```python
from build123d import *

# Parameters (mm, degrees)
SKETCH1_W            = 90
SKETCH1_H            = 70
BOSS_EXTRUDE1_DEPTH  = 10
FILLET1_R            = 4
SHELL1_T             = -2
SKETCH2_W            = 1
SKETCH2_H            = 15
BOSS_EXTRUDE2_DEPTH  = 1
SKETCH3_W            = 0.9
SKETCH3_H            = 15
BOSS_EXTRUDE3_DEPTH  = 0.9
SKETCH4_W            = 0.8
SKETCH4_H            = 15
BOSS_EXTRUDE4_DEPTH  = 0.8
SKETCH5_W            = 0.7
SKETCH5_H            = 15
BOSS_EXTRUDE5_DEPTH  = 0.7
SKETCH6_W            = 0.6
SKETCH6_H            = 15
BOSS_EXTRUDE6_DEPTH  = 0.6
SKETCH7_W            = 0.5
SKETCH7_H            = 15
BOSS_EXTRUDE7_DEPTH  = 0.5
SKETCH8_W            = 0.4
SKETCH8_H            = 15
BOSS_EXTRUDE8_DEPTH  = 0.4
SKETCH9_W            = 0.3
SKETCH9_H            = 15
BOSS_EXTRUDE9_DEPTH  = 0.3
SKETCH10_W           = 0.2
SKETCH10_H           = 15
BOSS_EXTRUDE10_DEPTH = 0.2
SKETCH11_W           = 0.1
SKETCH11_H           = 15
BOSS_EXTRUDE11_DEPTH = 0.1
SKETCH12_W           = 0.075
SKETCH12_H           = 15
BOSS_EXTRUDE12_DEPTH = 0.075
SKETCH14_W           = 0.05
SKETCH14_H           = 15
BOSS_EXTRUDE13_DEPTH = 0.05
SKETCH15_W           = 1
SKETCH15_H           = 15
BOSS_EXTRUDE14_DEPTH = 2
SKETCH17_W           = 0.9
SKETCH17_H           = 15
BOSS_EXTRUDE15_DEPTH = 1.8
SKETCH18_W           = 0.8
SKETCH18_H           = 15
BOSS_EXTRUDE16_DEPTH = 1.6
SKETCH19_W           = 0.7
SKETCH19_H           = 15
BOSS_EXTRUDE17_DEPTH = 1.4
SKETCH20_W           = 0.6
SKETCH20_H           = 15
BOSS_EXTRUDE18_DEPTH = 1.2
SKETCH21_W           = 0.5
SKETCH21_H           = 15
BOSS_EXTRUDE19_DEPTH = 1
SKETCH22_W           = 0.4
SKETCH22_H           = 15
BOSS_EXTRUDE20_DEPTH = 0.8
SKETCH23_W           = 0.3
SKETCH23_H           = 15
BOSS_EXTRUDE21_DEPTH = 0.6
SKETCH24_W           = 0.2
SKETCH24_H           = 15
BOSS_EXTRUDE22_DEPTH = 0.4
SKETCH25_W           = 0.1
SKETCH25_H           = 15
BOSS_EXTRUDE23_DEPTH = 0.2
SKETCH27_W           = 0.075
SKETCH27_H           = 15
BOSS_EXTRUDE24_DEPTH = 0.15
SKETCH28_W           = 0.05
SKETCH28_H           = 15
BOSS_EXTRUDE25_DEPTH = 0.1


with BuildPart() as part:
    # Sketch1 → Boss-Extrude1 (new body)
    with BuildSketch(Plane.XY):
        with Locations((45, 35)):
            Rectangle(SKETCH1_W, SKETCH1_H)
    extrude(amount=BOSS_EXTRUDE1_DEPTH)

    # Fillet1
    fillet1_edges = [part.edges().sort_by_distance(p)[0] for p in [
        (0, 70, 5),
        (90, 70, 5),
        (90, 0, 5),
        (0, 0, 5),
    ]]
    fillet(fillet1_edges, radius=FILLET1_R)

    # Shell1
    shell1_openings = [part.faces().sort_by_distance(p)[0] for p in [
        (45, 35, 10),
    ]]
    offset(amount=SHELL1_T, openings=shell1_openings, kind=Kind.INTERSECTION)

    # Sketch2 → Boss-Extrude2 (add)
    with BuildSketch(Plane.XY.offset(2)):
        with Locations((16.1, 50.5)):
            Rectangle(SKETCH2_W, SKETCH2_H)
    extrude(amount=BOSS_EXTRUDE2_DEPTH)

    # Sketch3 → Boss-Extrude3 (add)
    with BuildSketch(Plane.XY.offset(2)):
        with Locations((22.05, 50.5)):
            Rectangle(SKETCH3_W, SKETCH3_H)
    extrude(amount=BOSS_EXTRUDE3_DEPTH)

    # Sketch4 → Boss-Extrude4 (add)
    with BuildSketch(Plane.XY.offset(2)):
        with Locations((27.9, 50.5)):
            Rectangle(SKETCH4_W, SKETCH4_H)
    extrude(amount=BOSS_EXTRUDE4_DEPTH)

    # Sketch5 → Boss-Extrude5 (add)
    with BuildSketch(Plane.XY.offset(2)):
        with Locations((33.65, 50.5)):
            Rectangle(SKETCH5_W, SKETCH5_H)
    extrude(amount=BOSS_EXTRUDE5_DEPTH)

    # Sketch6 → Boss-Extrude6 (add)
    with BuildSketch(Plane.XY.offset(2)):
        with Locations((39.3, 50.5)):
            Rectangle(SKETCH6_W, SKETCH6_H)
    extrude(amount=BOSS_EXTRUDE6_DEPTH)

    # Sketch7 → Boss-Extrude7 (add)
    with BuildSketch(Plane.XY.offset(2)):
        with Locations((44.85, 50.5)):
            Rectangle(SKETCH7_W, SKETCH7_H)
    extrude(amount=BOSS_EXTRUDE7_DEPTH)

    # Sketch8 → Boss-Extrude8 (add)
    with BuildSketch(Plane.XY.offset(2)):
        with Locations((50.3, 50.5)):
            Rectangle(SKETCH8_W, SKETCH8_H)
    extrude(amount=BOSS_EXTRUDE8_DEPTH)

    # Sketch9 → Boss-Extrude9 (add)
    with BuildSketch(Plane.XY.offset(2)):
        with Locations((55.25, 50.5)):
            Rectangle(SKETCH9_W, SKETCH9_H)
    extrude(amount=BOSS_EXTRUDE9_DEPTH)

    # Sketch10 → Boss-Extrude10 (add)
    with BuildSketch(Plane.XY.offset(2)):
        with Locations((60.5, 50.5)):
            Rectangle(SKETCH10_W, SKETCH10_H)
    extrude(amount=BOSS_EXTRUDE10_DEPTH)

    # Sketch11 → Boss-Extrude11 (add)
    with BuildSketch(Plane.XY.offset(2)):
        with Locations((65.65, 50.5)):
            Rectangle(SKETCH11_W, SKETCH11_H)
    extrude(amount=BOSS_EXTRUDE11_DEPTH)

    # Sketch12 → Boss-Extrude12 (add)
    with BuildSketch(Plane.XY.offset(2)):
        with Locations((70.7375, 50.5)):
            Rectangle(SKETCH12_W, SKETCH12_H)
    extrude(amount=BOSS_EXTRUDE12_DEPTH)

    # Sketch14 → Boss-Extrude13 (add)
    with BuildSketch(Plane.XY.offset(2)):
        with Locations((75.8, 50.5)):
            Rectangle(SKETCH14_W, SKETCH14_H)
    extrude(amount=BOSS_EXTRUDE13_DEPTH)

    # Sketch15 → Boss-Extrude14 (add)
    with BuildSketch(Plane.XY.offset(2)):
        with Locations((16.1, 18.013180638)):
            Rectangle(SKETCH15_W, SKETCH15_H)
    extrude(amount=BOSS_EXTRUDE14_DEPTH)

    # Sketch17 → Boss-Extrude15 (add)
    with BuildSketch(Plane.XY.offset(2)):
        with Locations((22.05, 18.013180638)):
            Rectangle(SKETCH17_W, SKETCH17_H)
    extrude(amount=BOSS_EXTRUDE15_DEPTH)

    # Sketch18 → Boss-Extrude16 (add)
    with BuildSketch(Plane.XY.offset(2)):
        with Locations((27.9, 18.013180638)):
            Rectangle(SKETCH18_W, SKETCH18_H)
    extrude(amount=BOSS_EXTRUDE16_DEPTH)

    # Sketch19 → Boss-Extrude17 (add)
    with BuildSketch(Plane.XY.offset(2)):
        with Locations((33.65, 18.013180638)):
            Rectangle(SKETCH19_W, SKETCH19_H)
    extrude(amount=BOSS_EXTRUDE17_DEPTH)

    # Sketch20 → Boss-Extrude18 (add)
    with BuildSketch(Plane.XY.offset(2)):
        with Locations((39.3, 18.013180638)):
            Rectangle(SKETCH20_W, SKETCH20_H)
    extrude(amount=BOSS_EXTRUDE18_DEPTH)

    # Sketch21 → Boss-Extrude19 (add)
    with BuildSketch(Plane.XY.offset(2)):
        with Locations((44.85, 18.013180638)):
            Rectangle(SKETCH21_W, SKETCH21_H)
    extrude(amount=BOSS_EXTRUDE19_DEPTH)

    # Sketch22 → Boss-Extrude20 (add)
    with BuildSketch(Plane.XY.offset(2)):
        with Locations((50.3, 18.013180638)):
            Rectangle(SKETCH22_W, SKETCH22_H)
    extrude(amount=BOSS_EXTRUDE20_DEPTH)

    # Sketch23 → Boss-Extrude21 (add)
    with BuildSketch(Plane.XY.offset(2)):
        with Locations((55.25, 18.013180638)):
            Rectangle(SKETCH23_W, SKETCH23_H)
    extrude(amount=BOSS_EXTRUDE21_DEPTH)

    # Sketch24 → Boss-Extrude22 (add)
    with BuildSketch(Plane.XY.offset(2)):
        with Locations((60.5, 18.013180638)):
            Rectangle(SKETCH24_W, SKETCH24_H)
    extrude(amount=BOSS_EXTRUDE22_DEPTH)

    # Sketch25 → Boss-Extrude23 (add)
    with BuildSketch(Plane.XY.offset(2)):
        with Locations((65.65, 18.013180638)):
            Rectangle(SKETCH25_W, SKETCH25_H)
    extrude(amount=BOSS_EXTRUDE23_DEPTH)

    # Sketch27 → Boss-Extrude24 (add)
    with BuildSketch(Plane.XY.offset(2)):
        with Locations((70.7375, 18.013180638)):
            Rectangle(SKETCH27_W, SKETCH27_H)
    extrude(amount=BOSS_EXTRUDE24_DEPTH)

    # Sketch28 → Boss-Extrude25 (add)
    with BuildSketch(Plane.XY.offset(2)):
        with Locations((75.8, 18.013180638)):
            Rectangle(SKETCH28_W, SKETCH28_H)
    extrude(amount=BOSS_EXTRUDE25_DEPTH)


solid = part.part
```
Geometry check sheet. Reference: the model listing, model coordinates, mm. A direction names the side the tool comes from. Give positions to 0.01 mm unless a question says otherwise; leave off trailing zeros. Order: outer loops, then holes, each group sorted by start corner. A loop starts at its lowest first (then second) coordinate and runs counter-clockwise, first axis right, second up.
1. Gauge pin test, flat end, axial feed: pin 1 Ø6 at (x, y) = (75, 61.5) entering from +Z. Record the tip position at first contact, or that the pin passes through.
2. Section check A-A, the plane z = 7. Enter the section's corners in (x, y).
3. Thickness scan on L1, parallel to Y at x = 46, z = 6; L2, parallel to X at y = 66, z = 4.75; L3, parallel to Z at x = 81.5, y = 5.5. Record the ranges inside material, lowest first.
4. Section check C-C, the plane x = 7. Enter the section's corners in (y, z).
5. Release check for a two-part mould opening along X. For faces 1 (the face through (88.797, 1.141, 5.07)), 2 (the face through (2, 35, 6)), 3 (the face through (44, 35, 0)) record: pulls with the +X half, pulls with the -X half, needs draft (parallel to the pull), parting line crosses it, or undercut.
6. Section check B-B, the plane y = 28.5. Enter the section's corners in (x, z).
7. Access from +Z, -Z, +X, -X, +Y, -Y to the whole of each face (thin tool, end or side, straight path). Record for faces 4 (the face through (88, 35, 6)), 5 (the face through (44, 70, 5)).
Values follow:
1. pin 1: stops at z = 2
2. outline: (0, 4) arc R4 ccw to (4, 0) - (86, 0) arc R4 ccw to (90, 4) - (90, 66) arc R4 ccw to (86, 70) - (4, 70) arc R4 ccw to (0, 66) - close; hole (2, 4) arc R2 ccw to (4, 2) - (86, 2) arc R2 ccw to (88, 4) - (88, 66) arc R2 ccw to (86, 68) - (4, 68) arc R2 ccw to (2, 66) - close
3. L1: y = 0 to 2, 68 to 70
3. L2: x = 0 to 2, 88 to 90
3. L3: z = 0 to 2
4. outline: (0, 0) - (70, 0) - (70, 10) - (68, 10) - (68, 2) - (2, 2) - (2, 10) - (0, 10) - close
5. face 1: pulls with the +X half
5. face 2: undercut
5. face 3: needs draft
6. outline: (0, 0) - (90, 0) - (90, 10) - (88, 10) - (88, 2) - (2, 2) - (2, 10) - (0, 10) - close
7. face 4: +Z
7. face 5: +Z, -Z, +X, -X, +Y
